Input: part model. Units: mm. Frame: model coordinates. A direction names the side the tool comes from. Give positions to 0.01 mm unless a question says otherwise; leave off trailing zeros. Write each loop counter-clockwise with the first axis right and the second up, starting at its lowest first coordinate (ties: lowest second). Pieces come first, ordered by that corner, then holes. Notation, with made-up numbers: (67.5, 51) - (115.5, 51) arc R14 ccw to (115.5, 75) - close; hole circle Ø10 at (71, 21.25). An arc over 180 degrees is marked (long way). Use a Markdown table: item, result. Add a question column.
1. Section query D-D, the plane x = -4.5. Return loops of the section in (y, z).
2. Material intervals for probe 1 along X at (y, z) = (11, -1.2); probe 2 along Y at (x, z) = (0, 1.45); probe 3 along Y at (x, z) = (1, 0.5), sorted ascending.
3. Section query B-B, the plane y = 11.5. Return loops of the section in (x, z), plus the area to 3 significant figures.
4. Set-up query: faces 5 (the flat face through (-8, 12, 0)), 6 (the flat face through (3, 12, 0)). Return all of +Z, -Z, +X, -X, +Y, -Y with unobstructed straight access to the full face (end or side cutting, diameter ignored); none if empty.
5. Section query A-A, the plane z = 0. Return loops of the section in (x, y).
6. Section query C-C, the plane x = 0. Return loops of the section in (y, z), plus the area to 3 significant figures.
7. Mould query, pull axis X, two halves, no side actions, for faces 1 (the flat face through (-3, 12, 0)), 2 (the flat face through (0, 7, 0)), 3 (the cylindrical face through (7.1, 0.86, -0.04)), 4 (the flat face through (-0.1, 6.7, 3)). Classes: released by +X, released by -X, zero draft, split by the parting line, or undercut.
```python
from build123d import *

# Parameters (mm, degrees)
SKETCH_1_W          = 16
SKETCH_1_H          = 6
EXTRUDE_1_DEPTH     = 7
SKETCH_3_R          = 1.5
EXTRUDE_2_DEPTH     = 8
SKETCH_3_2_R        = 1.5
CUT_EXTRUDE_2_DEPTH = 3
SKETCH_9_R          = 1.5
CUT_EXTRUDE_3_DEPTH = 10
FILLET_4_R          = 3
FILLET_5_R          = 3


with BuildPart() as part:
    # 草图1 → 凸台-拉伸1 (new body)
    with BuildSketch(Plane(origin=(0, 0, 0), x_dir=(1, 0, 0), z_dir=(0, 1, 0))):
        Rectangle(SKETCH_1_W, SKETCH_1_H)
    extrude(amount=EXTRUDE_1_DEPTH)

    # 草图3 → 凸台-拉伸2 (add, symmetric)
    with BuildSketch(Plane.ZY):
        with BuildLine():
            Line((3, 7), (-3, 7))
            Line((-3, 7), (-3, 17))
            ThreePointArc((-3, 17), (0, 20), (3, 17))
            Line((3, 17), (3, 7))
        make_face()
        with Locations((-0.000581651, 16.923736161)):
            Circle(SKETCH_3_R, mode=Mode.SUBTRACT)
    extrude(amount=EXTRUDE_2_DEPTH, both=True)

    # 草图3<2> → 切除-拉伸2 (cut, symmetric)
    with BuildSketch(Plane.ZY):
        with BuildLine():
            Line((3, 7), (-3, 7))
            Line((-3, 7), (-3, 17))
            ThreePointArc((-3, 17), (0, 20), (3, 17))
            Line((3, 17), (3, 7))
        make_face()
        with Locations((-0.000581651, 16.923736161)):
            Circle(SKETCH_3_2_R, mode=Mode.SUBTRACT)
    extrude(amount=CUT_EXTRUDE_2_DEPTH, both=True, mode=Mode.SUBTRACT)

    # 草图9 → 切除-拉伸3 (cut)
    with BuildSketch(Plane.XY.offset(5)):
        with Locations((0, 3.5)):
            Circle(SKETCH_9_R)
    extrude(amount=-CUT_EXTRUDE_3_DEPTH, mode=Mode.SUBTRACT)

    # 圆角4
    fillet_4_edges = [part.edges().sort_by_distance(p)[0] for p in [
        (8, 0, 0),
    ]]
    fillet(fillet_4_edges, radius=FILLET_4_R)

    # 圆角5
    fillet_5_edges = [part.edges().sort_by_distance(p)[0] for p in [
        (-8, 0, 0),
    ]]
    fillet(fillet_5_edges, radius=FILLET_5_R)


solid = part.part
```
Result sheet:
| question | item | result |
|---|---|---|
| 1 | outline | (0, -3) - (17, -3) arc R3 ccw to (17, 3) - (0, 3) - close; hole circle Ø3 at (16.92, 0) |
| 2 | probe 1 | x = -8 to -3, 3 to 8 |
| 2 | probe 2 | y = 0 to 2, 5 to 7 |
| 2 | probe 3 | y = 0 to 2.38, 4.62 to 7 |
| 3 | outline | (-8, -3) - (-3, -3) - (-3, 3) - (-8, 3) - close; (3, -3) - (8, -3) - (8, 3) - (3, 3) - close |
| 3 | area | 60.0 mm² |
| 4 | face 5 | +Z, -Z, -X, +Y, -Y |
| 4 | face 6 | +Z, -Z, +Y |
| 5 | outline | (-8, 3) arc R3 ccw to (-5, 0) - (5, 0) arc R3 ccw to (8, 3) - (8, 15.42) - (3, 15.42) - (3, 7) - (-3, 7) - (-3, 15.42) - (-8, 15.42) - close; (-8, 18.42) - (-3, 18.42) - (-3, 20) - (-8, 20) - close; (3, 18.42) - (8, 18.42) - (8, 20) - (3, 20) - close; hole circle Ø3 at (0, 3.5) |
| 6 | outline | (0, -3) - (2, -3) - (2, 3) - (0, 3) - close; (5, -3) - (7, -3) - (7, 3) - (5, 3) - close |
| 6 | area | 24.0 mm² |
| 7 | face 1 | undercut |
| 7 | face 2 | undercut |
| 7 | face 3 | released by +X |
| 7 | face 4 | zero draft |
